```python
from build123d import *

# Parameters (mm, degrees)
BOSS_EXTRUDE1_DEPTH = 10
SKETCH3_R           = 3.1
CUT_EXTRUDE1_DEPTH  = 10
CUT_EXTRUDE4_DEPTH  = 10
BOSS_EXTRUDE2_DEPTH = 10
SKETCH9_R           = 5
CUT_EXTRUDE5_DEPTH  = 3.5


with BuildPart() as part:
    # Sketch1 → Boss-Extrude1 (new body)
    with BuildSketch(Plane.YZ):
        Polygon((122.8604, 156.33104), (123.6529, 156.40531), (124.8827, 156.22038), (126.9389, 155.34362), (126.9389, 153.95038), (124.8827, 153.07362), (123.6529, 152.88869), (122.8604, 152.96296), (122.5013, 150.69576), (123.278, 150.5215), (124.3904, 149.9656), (126.075, 148.49636), (125.6445, 147.1713), (123.418, 146.97285), (122.1913, 147.17699), (121.4605, 147.49252), (120.4184, 145.44725), (121.1032, 145.04152), (121.9894, 144.1691), (123.1376, 142.2512), (122.3186, 141.124), (120.1398, 141.6233), (119.0362, 142.1965), (118.4387, 142.7224), (116.8156, 141.0993), (117.3415, 140.5018), (117.9147, 139.3982), (118.414, 137.2194), (117.2868, 136.4004), (115.3689, 137.5486), (114.49648, 138.4348), (114.09075, 139.1196), (112.04548, 138.0775), (112.36101, 137.3467), (112.56515, 136.12), (112.3667, 133.8935), (111.04164, 133.463), (109.5724, 135.1476), (109.0165, 136.26), (108.84224, 137.0367), (106.57504, 136.6776), (106.64931, 135.8851), (106.46438, 134.6553), (105.58762, 132.5991), (104.19438, 132.5991), (103.31762, 134.6553), (103.13269, 135.8851), (103.20696, 136.6776), (100.93976, 137.0367), (100.7655, 136.26), (100.2096, 135.1476), (98.74036, 133.463), (97.4153, 133.8935), (97.21685, 136.12), (97.42099, 137.3467), (97.73652, 138.0775), (95.69125, 139.1196), (95.28552, 138.4348), (94.4131, 137.5486), (92.4952, 136.4004), (91.368, 137.2194), (91.8673, 139.3982), (92.4405, 140.5018), (92.9664, 141.0993), (91.3433, 142.7224), (90.7458, 142.1965), (89.6422, 141.6233), (87.4634, 141.124), (86.6444, 142.2512), (87.7926, 144.1691), (88.6788, 145.04152), (89.3636, 145.44725), (88.3215, 147.49252), (87.5907, 147.17699), (86.364, 146.97285), (84.1375, 147.1713), (83.707, 148.49636), (85.3916, 149.9656), (86.504, 150.5215), (87.2807, 150.69576), (86.9216, 152.96296), (86.1291, 152.88869), (84.8993, 153.07362), (82.8431, 153.95038), (82.8431, 155.34362), (84.8993, 156.22038), (86.1291, 156.40531), (86.9216, 156.33104), (87.2807, 158.59824), (86.504, 158.7725), (85.3916, 159.3284), (83.707, 160.79764), (84.1375, 162.1227), (86.364, 162.32115), (87.5907, 162.11701), (88.3215, 161.80148), (89.3636, 163.84675), (88.6788, 164.25248), (87.7926, 165.1249), (86.6444, 167.0428), (87.4634, 168.17), (89.6422, 167.6707), (90.7458, 167.0975), (91.3433, 166.5716), (92.9664, 168.1947), (92.4405, 168.7922), (91.8673, 169.8958), (91.368, 172.0746), (92.4952, 172.8936), (94.4131, 171.7454), (95.28552, 170.8592), (95.69125, 170.1744), (97.73652, 171.2165), (97.42099, 171.9473), (97.21685, 173.174), (97.4153, 175.4005), (98.74036, 175.831), (100.2096, 174.1464), (100.7655, 173.034), (100.93976, 172.2573), (103.20696, 172.6164), (103.13269, 173.4089), (103.31762, 174.6387), (104.19438, 176.6949), (105.58762, 176.6949), (106.46438, 174.6387), (106.64931, 173.4089), (106.57504, 172.6164), (108.84224, 172.2573), (109.0165, 173.034), (109.5724, 174.1464), (111.04164, 175.831), (112.3667, 175.4005), (112.56515, 173.174), (112.36101, 171.9473), (112.04548, 171.2165), (114.09075, 170.1744), (114.49648, 170.8592), (115.3689, 171.7454), (117.2868, 172.8936), (118.414, 172.0746), (117.9147, 169.8958), (117.3415, 168.7922), (116.8156, 168.1947), (118.4387, 166.5716), (119.0362, 167.0975), (120.1398, 167.6707), (122.3186, 168.17), (123.1376, 167.0428), (121.9894, 165.1249), (121.1032, 164.25248), (120.4184, 163.84675), (121.4605, 161.80148), (122.1913, 162.11701), (123.418, 162.32115), (125.6445, 162.1227), (126.075, 160.79764), (124.3904, 159.3284), (123.278, 158.7725), (122.5013, 158.59824), align=None)
    extrude(amount=BOSS_EXTRUDE1_DEPTH)

    # Sketch3 → Cut-Extrude1 (cut)
    with BuildSketch(Plane.YZ.offset(10)):
        with Locations(Location((104.891, 154.647, 0), (0, 0, 270))):
            Circle(SKETCH3_R)
    extrude(amount=-CUT_EXTRUDE1_DEPTH, mode=Mode.SUBTRACT)

    # Sketch5 → Cut-Extrude4 (cut)
    with BuildSketch(Plane.YZ.offset(10)):
        with BuildLine():
            Line((92.9664, 168.1947), (90.294048938, 171.230794333))
            ThreePointArc((90.294048938, 171.230794333), (83.487848916, 149.169926106), (100.054261516, 133.090117674))
            Line((100.054261516, 133.090117674), (100.93976, 137.0367))
            ThreePointArc((100.93976, 137.0367), (87.406270735, 150.172651628), (92.9664, 168.1947))
        make_face()
    extrude(amount=-CUT_EXTRUDE4_DEPTH, mode=Mode.SUBTRACT)


with BuildPart() as cut_extrude4_kept_piece:
    # of the separate pieces the step leaves, the one the design keeps (cut_extrude4_pieces_kept)
    add(part.part.solids().sort_by_distance((0, 122.8604, 156.33104))[0])

    # Sketch8 → Boss-Extrude2 (add)
    with BuildSketch(Plane(origin=(0, 0, 0), x_dir=(0, -1, 0), z_dir=(-1, 0, 0))):
        with BuildLine():
            Line((-101.292796156, 158.234170992), (-100.358785712, 141.250463774))
            Line((-100.358785712, 141.250463774), (-42.28117848, 138.036732938))
            Line((-42.28117848, 138.036732938), (-33.120005133, 161.580447331))
            Line((-33.120005133, 161.580447331), (-33.120005133, 170.304878432))
            Line((-33.120005133, 170.304878432), (-46.164559873, 171.026700315))
            ThreePointArc((-46.164559873, 171.026700315), (-59.339432356, 159.173287387), (-71.126053545, 172.407947335))
            Line((-71.126053545, 172.407947335), (-82.067282372, 173.013381445))
            add(Edge.make_bspline(
                [(-101.292796156, 158.234170992), (-79.754841913, 159.418639963), (-82.067282372, 173.013381445)],
                knots=[4.799124848, 4.799124848, 4.799124848, 6.390352549, 6.390352549, 6.390352549], degree=2, weights=[1, 0.699846429, 1]))
        make_face()
    extrude(amount=-BOSS_EXTRUDE2_DEPTH)

    # Sketch9 → Cut-Extrude5 (cut)
    with BuildSketch(Plane.YZ.offset(10)):
        with Locations(Location((104.891, 154.647, 0), (0, 0, 270))):
            Circle(SKETCH9_R)
    extrude(amount=-CUT_EXTRUDE5_DEPTH, mode=Mode.SUBTRACT)


solid = cut_extrude4_kept_piece.part
```
Check sheet for the modelled part. Datum: model origin and axes. Units: mm. A direction names the side the tool comes from. Give positions to 0.01 mm unless a question says otherwise; leave off trailing zeros. Loops run counter-clockwise (first coordinate to the right, second up) from the corner with the lowest first, then second, coordinate; pieces in that order, holes last. Notation, with made-up numbers: (-26, 74) - (22, 74) arc R11 cw to (22, 92) - close; hole circle Ø11 at (54.5, 8.25). An arc over 180 degrees is marked (long way). One line per question, with ' | ' between items. Start each with the question number.
1. Draft check along Y on faces 4 (the flat face through (5, 33.12, 166)), 5 (the flat face through (4.93, 112.467, 135.022)), 6 (the cylindrical face through (5.07, 94.45, 139.925)). Enter one of: released by +Y, released by -Y, zero draft, split by the parting line, or undercut.
2. Gauge pin test, flat ends, axial feed: pin 1 Ø1 at (x, y) = (9, 55.5) entering from +Z; pin 2 Ø13 at (y, z) = (104.891, 154.647) entering from -X; pin 3 Ø5.5 at (y, z) = (104.891, 154.647) entering from -X (3 decimals); pin 4 Ø1 at (x, y) = (7, 94.5) entering from +Z. Record the tip position at first contact, or that the pin passes through.
3. Set-up check for faces 1 (the flat face through (4.93, 106.03, 133.64)), 2 (the flat face through (4.93, 116.31, 172.31)), 3 (the flat face through (4.93, 92.14, 167.37)): record each of +Z, -Z, +X, -X, +Y, -Y from which the full face is reachable in a straight line by a thin tool's end or side.
4. Cross-section at B-B, the plane y = 51. Enter the section's corners in (x, z).
5. Cross-section at A-A, the plane y = 61.5. Enter the section's corners in (x, z), plus the area to 3 significant figures.
6. Material ranges on line 1 along Y through (x, z) = (6.25, 165); line 2 along Z through (x, y) = (7.5, 121); line 3 along Y through (x, z) = (1.75, 168.5), recorded low to high. Write a range as [from, to].
Check result:
1) face 4: released by -Y | face 5: released by +Y | face 6: undercut
2) pin 1: stops at z = 159.7 | pin 2: stops at x = 0 | pin 3: passes through | pin 4: stops at z = 171.99
3) face 1: -Z, +X, -X | face 2: +Z, +X, -X | face 3: +X, -X
4) outline: (0, 138.52) - (10, 138.52) - (10, 161.77) - (0, 161.77) - close
5) outline: (0, 139.1) - (10, 139.1) - (10, 159.48) - (0, 159.48) - close | area: 204 mm2
6) line 1: y = [33.12, 48.07], [69.23, 84.68], [90.11, 121.86] | line 2: z = [141.43, 145.1], [146.59, 162.71], [164.19, 167.87] | line 3: y = [33.12, 46.55], [70.74, 82.51], [92.7, 117.08]
